from build123d import *

# Parameters (mm, degrees)
SKETCH_1_W          = 100
SKETCH_1_H          = 100
EXTRUDE_1_DEPTH     = 8
SKETCH_2_W          = 60
SKETCH_2_H          = 60
EXTRUDE_2_DEPTH     = 2
SKETCH_3_R          = 3
EXTRUDE_3_DEPTH     = 40
SKETCH_4_R          = 4
CUT_EXTRUDE_1_DEPTH = 4
SKETCH_5_R          = 2.25
CUT_EXTRUDE_2_DEPTH = 82.240384046


with BuildPart() as part:
    # 草图1 → 凸台-拉伸1 (new body)
    with BuildSketch(Plane.XY):
        Rectangle(SKETCH_1_W, SKETCH_1_H)
    extrude(amount=EXTRUDE_1_DEPTH)

    # 草图2 → 凸台-拉伸2 (add)
    with BuildSketch(Plane.XY):
        Rectangle(SKETCH_2_W, SKETCH_2_H)
    extrude(amount=-EXTRUDE_2_DEPTH)

    # 草图3 → 凸台-拉伸3 (add)
    with BuildSketch(Plane.XY.offset(8)):
        with Locations((-40, -30)):
            Circle(SKETCH_3_R)
        with Locations((-40, -20)):
            Circle(SKETCH_3_R)
        with Locations((-40, -10)):
            Circle(SKETCH_3_R)
        with Locations((-40, 0)):
            Circle(SKETCH_3_R)
        with Locations((-40, 10)):
            Circle(SKETCH_3_R)
        with Locations((-40, 20)):
            Circle(SKETCH_3_R)
        with Locations((-40, 30)):
            Circle(SKETCH_3_R)
        with Locations((-30, -40)):
            Circle(SKETCH_3_R)
        with Locations((-30, -30)):
            Circle(SKETCH_3_R)
        with Locations((-30, -20)):
            Circle(SKETCH_3_R)
        with Locations((-30, -10)):
            Circle(SKETCH_3_R)
        with Locations((-30, 0)):
            Circle(SKETCH_3_R)
        with Locations((-30, 10)):
            Circle(SKETCH_3_R)
        with Locations((-30, 20)):
            Circle(SKETCH_3_R)
        with Locations((-30, 30)):
            Circle(SKETCH_3_R)
        with Locations((-30, 40)):
            Circle(SKETCH_3_R)
        with Locations((-20, -40)):
            Circle(SKETCH_3_R)
        with Locations((-20, -30)):
            Circle(SKETCH_3_R)
        with Locations((-20, -20)):
            Circle(SKETCH_3_R)
        with Locations((-20, -10)):
            Circle(SKETCH_3_R)
        with Locations((-20, 0)):
            Circle(SKETCH_3_R)
        with Locations((-20, 10)):
            Circle(SKETCH_3_R)
        with Locations((-20, 20)):
            Circle(SKETCH_3_R)
        with Locations((-20, 30)):
            Circle(SKETCH_3_R)
        with Locations((-20, 40)):
            Circle(SKETCH_3_R)
        with Locations((-10, -40)):
            Circle(SKETCH_3_R)
        with Locations((-10, -30)):
            Circle(SKETCH_3_R)
        with Locations((-10, -20)):
            Circle(SKETCH_3_R)
        with Locations((-10, -10)):
            Circle(SKETCH_3_R)
        with Locations((-10, 0)):
            Circle(SKETCH_3_R)
        with Locations((-10, 10)):
            Circle(SKETCH_3_R)
        with Locations((-10, 20)):
            Circle(SKETCH_3_R)
        with Locations((-10, 30)):
            Circle(SKETCH_3_R)
        with Locations((-10, 40)):
            Circle(SKETCH_3_R)
        with Locations((0, -40)):
            Circle(SKETCH_3_R)
        with Locations((0, -30)):
            Circle(SKETCH_3_R)
        with Locations((0, -20)):
            Circle(SKETCH_3_R)
        with Locations((0, -10)):
            Circle(SKETCH_3_R)
        Circle(SKETCH_3_R)
        with Locations((0, 10)):
            Circle(SKETCH_3_R)
        with Locations((0, 20)):
            Circle(SKETCH_3_R)
        with Locations((0, 30)):
            Circle(SKETCH_3_R)
        with Locations((0, 40)):
            Circle(SKETCH_3_R)
        with Locations((10, -40)):
            Circle(SKETCH_3_R)
        with Locations((10, -30)):
            Circle(SKETCH_3_R)
        with Locations((10, -20)):
            Circle(SKETCH_3_R)
        with Locations((10, -10)):
            Circle(SKETCH_3_R)
        with Locations((10, 0)):
            Circle(SKETCH_3_R)
        with Locations((10, 10)):
            Circle(SKETCH_3_R)
        with Locations((10, 20)):
            Circle(SKETCH_3_R)
        with Locations((10, 30)):
            Circle(SKETCH_3_R)
        with Locations((10, 40)):
            Circle(SKETCH_3_R)
        with Locations((20, -40)):
            Circle(SKETCH_3_R)
        with Locations((20, -30)):
            Circle(SKETCH_3_R)
        with Locations((20, -20)):
            Circle(SKETCH_3_R)
        with Locations((20, -10)):
            Circle(SKETCH_3_R)
        with Locations((20, 0)):
            Circle(SKETCH_3_R)
        with Locations((20, 10)):
            Circle(SKETCH_3_R)
        with Locations((20, 20)):
            Circle(SKETCH_3_R)
        with Locations((20, 30)):
            Circle(SKETCH_3_R)
        with Locations((20, 40)):
            Circle(SKETCH_3_R)
        with Locations((30, -40)):
            Circle(SKETCH_3_R)
        with Locations((30, -30)):
            Circle(SKETCH_3_R)
        with Locations((30, -20)):
            Circle(SKETCH_3_R)
        with Locations((30, -10)):
            Circle(SKETCH_3_R)
        with Locations((30, 0)):
            Circle(SKETCH_3_R)
        with Locations((30, 10)):
            Circle(SKETCH_3_R)
        with Locations((30, 20)):
            Circle(SKETCH_3_R)
        with Locations((30, 30)):
            Circle(SKETCH_3_R)
        with Locations((30, 40)):
            Circle(SKETCH_3_R)
        with Locations((40, -30)):
            Circle(SKETCH_3_R)
        with Locations((40, -20)):
            Circle(SKETCH_3_R)
        with Locations((40, -10)):
            Circle(SKETCH_3_R)
        with Locations((40, 0)):
            Circle(SKETCH_3_R)
        with Locations((40, 10)):
            Circle(SKETCH_3_R)
        with Locations((40, 20)):
            Circle(SKETCH_3_R)
        with Locations((40, 30)):
            Circle(SKETCH_3_R)
    extrude(amount=EXTRUDE_3_DEPTH)

    # 草图4 → 切除-拉伸1 (cut)
    with BuildSketch(Plane.XY.offset(8)):
        with Locations((-40, -40)):
            Circle(SKETCH_4_R)
        with Locations((-40, 40)):
            Circle(SKETCH_4_R)
        with Locations((40, -40)):
            Circle(SKETCH_4_R)
        with Locations((40, 40)):
            Circle(SKETCH_4_R)
    extrude(amount=-CUT_EXTRUDE_1_DEPTH, mode=Mode.SUBTRACT)

    # 草图5 → 切除-拉伸2 (cut, through all)
    with BuildSketch(Plane.XY.offset(8)):
        with Locations((-40, -40)):
            Circle(SKETCH_5_R)
        with Locations((-40, 40)):
            Circle(SKETCH_5_R)
        with Locations((40, -40)):
            Circle(SKETCH_5_R)
        with Locations((40, 40)):
            Circle(SKETCH_5_R)
    extrude(amount=-CUT_EXTRUDE_2_DEPTH, mode=Mode.SUBTRACT)


solid = part.part
Could you check a few things on this model? Use its own coordinates, in mm. A direction names the side the tool comes from. Coordinates: 2 decimals unless noted, no trailing zeros. Write each loop counter-clockwise with the first axis right and the second up, starting at its lowest first coordinate (ties: lowest second). Pieces come first, ordered by that corner, then holes. Notation, with made-up numbers: M 69,-14.75 L 77,-14.75 A22 cw 77,-4.75 Z; hole C 46.25,28 d11. An arc over 180 degrees is marked long. One line per question, with ' | ' between items.
1) For faces 4 (the face through (20, 30, 48)), 5 (the face through (-33, -20, 28)), which set-ups out of +Z, -Z, +X, -X, +Y, -Y let a thin tool reach every point of the face, with its end or its side?
Checks:
face 4: +Z, +X, -X, +Y, -Y | face 5: +Z
2) I need wall thicknesses on probe 1 along Y at (x, z) = (-40, 0.9); probe 2 along Z at (x, y) = (-3.5, -10); probe 3 along Z at (x, y) = (33, 1). Which ranges of each line are inside material? Lowest first, please. Write a range as [from, to].
Checks:
probe 1: [-50, -42.25], [-37.75, 37.75], [42.25, 50] | probe 2: [-2, 8] | probe 3: [0, 8]
3) If we mould it in two halves opening along X, with no side actions, what happens to faces 1 (the face through (42, 38, 4)), 2 (the face through (-50, -1, 4)), 3 (the face through (0, -30, 48))? For each: released by +X, released by -X, zero draft, split by the parting line, or undercut.
Checks:
face 1: undercut | face 2: released by -X | face 3: zero draft
4) For pin 1 Ø5 at (x, y) = (40, 40) entering from +Z; pin 2 Ø3.5 at (x, y) = (-40, 40) entering from +Z; pin 3 Ø9 at (x, y) = (-41.5, -40) entering from +Z; pin 4 Ø1.5 at (y, z) = (-20, 39) entering from -X, each with a flat end and sliding along its axis, tell me the tip position at first contact or that it passes through.
Checks:
pin 1: z = 4 | pin 2: through | pin 3: z = 8 | pin 4: x = -43
5) Imagine slicing it at A-A, the plane y = -40. Give the number of separate pieces and of enclosed holes in the cut face, and give its area (3 significant figures).
Checks:
separate pieces: 3 | enclosed holes: 0 | area: 2,380 mm²
6) Imagine slicing it at C-C, the plane x = 15.5. Write out the boundary of the cut face in (y, z), and give its area (3 significant figures).
Checks:
outline: M -50,0 L -30,0 L -30,-2 L 30,-2 L 30,0 L 50,0 L 50,8 L -50,8 Z | area: 920 mm²
